```python
from build123d import *

# Parameters (mm, degrees)
CHANFREIN1_SIZE         = 1
CHANFREIN1_SIZE2        = 1.732050808
ESQUISSE3_W             = 48.532957324
ESQUISSE3_H             = 12
ENL_V_MAT_EXTRU_1_DEPTH = 1
ESQUISSE4_OUTSIDE_W     = 40.012
ESQUISSE4_OUTSIDE_H     = 40.012
ESQUISSE4_OUTSIDE_R     = 4.5
ENL_V_MAT_EXTRU_2_DEPTH = 20
ESQUISSE5_W             = 37.366082186
ESQUISSE5_H             = 10
ENL_V_MAT_EXTRU_3_DEPTH = 1.5
CHANFREIN2_SIZE         = 0.5
CHANFREIN3_SIZE         = 0.3


with BuildPart() as part:
    # Esquisse1 → Révolution1 (revolve)
    with BuildSketch(Plane.XY, mode=Mode.PRIVATE) as r_volution1_sk:
        Polygon((5, 73.557112482), (5, -1.442887518), (8.25, -1.442887518), (8.25, -20.442887518), (5, -20.442887518), (5, -31.442887518), (0, -31.442887518), (0, 73.557112482), align=None)
    revolve(r_volution1_sk.sketch.rotate(Axis((0, 73.557112482, 0), (0, -1, 0)), 180), axis=Axis((0, 73.557112482, 0), (0, -1, 0)))  # turned: the seam where the file's is

    # Chanfrein1
    chanfrein1_edges = [part.edges().sort_by_distance(p)[0] for p in [
        (5, -31.442887518, 0),
    ]]
    chanfrein1_side = [part.faces().sort_by_distance(p)[0] for p in [
        (0, -31.442887518, 0),
    ]]
    chamfer(chanfrein1_edges, length=CHANFREIN1_SIZE, length2=CHANFREIN1_SIZE2, reference=chanfrein1_side[0])

    # Esquisse3 → Enlèv. mat.-Extru.1 (cut)
    with BuildSketch(Plane.XY.offset(5)):
        with Locations((0, 37.557112482)):
            Rectangle(ESQUISSE3_W, ESQUISSE3_H)
    extrude(amount=-ENL_V_MAT_EXTRU_1_DEPTH, mode=Mode.SUBTRACT)

    # Esquisse4 outside → Enlèv. mat.-Extru.2 (cut)
    with BuildSketch(Plane(origin=(0, 73.557112482, 0), x_dir=(1, 0, 0), z_dir=(0, 1, 0))):
        Rectangle(ESQUISSE4_OUTSIDE_W, ESQUISSE4_OUTSIDE_H)
        with Locations(Location((0, 0, 0), (0, 0, 180))):  # turned: the seam where the file's is
            Circle(ESQUISSE4_OUTSIDE_R, mode=Mode.SUBTRACT)
    extrude(amount=-ENL_V_MAT_EXTRU_2_DEPTH, mode=Mode.SUBTRACT)

    # Esquisse5 → Enlèv. mat.-Extru.3 (cut)
    with BuildSketch(Plane.XY.offset(5)):
        with Locations((0, 63.557112482)):
            Rectangle(ESQUISSE5_W, ESQUISSE5_H)
    extrude(amount=-ENL_V_MAT_EXTRU_3_DEPTH, mode=Mode.SUBTRACT)

    # Chanfrein2
    chanfrein2_edges = [part.edges().sort_by_distance(p)[0] for p in [
        (4.5, 73.557112482, 0),
    ]]
    chamfer(chanfrein2_edges, length=CHANFREIN2_SIZE)

    # Chanfrein3
    chanfrein3_edges = [part.edges().sort_by_distance(p)[0] for p in [
        (8.25, -1.442887518, 0),
        (8.25, -20.442887518, 0),
    ]]
    chamfer(chanfrein3_edges, length=CHANFREIN3_SIZE)


solid = part.part
```
Input: part model. Units: mm. Frame: model coordinates. A direction names the side the tool comes from. Give positions to 0.01 mm unless a question says otherwise; leave off trailing zeros. Order: outer loops, then holes, each group sorted by start corner. A loop starts at its lowest first (then second) coordinate and runs counter-clockwise, first axis right, second up. Notation, with made-up numbers: (-23, 55) - (28, 55) arc R23 ccw to (28, 91) - close; hole circle Ø3 at (-2.75, 18.25). An arc over 180 degrees is marked (long way). One line per item, written item: value.
1. Reachability of faces 5 (the face through (0, 64, 3.5)), 6 (the face through (0.98, 63.44, -4.39)), 7 (the face through (-5.2, -20.443, -0.1)) from +Z, -Z, +X, -X, +Y, -Y: full face, straight path, thin tool, end or side. Return the list, or none.
Determined:
face 5: +Z, +X, -X
face 6: +Y
face 7: -Y
2. Pin query (flat end, axial travel): pin 1 Ø0.5 at (x, z) = (0.5, 4.5) entering from -Y; pin 2 Ø1 at (x, y) = (-3.5, 8.5) entering from +Z; pin 3 Ø4 at (x, z) = (4, 3.5) entering from +Y; pin 4 Ø8 at (x, y) = (1.5, 18) entering from +Z. Return the tip coordinate at first contact, or that it passes through.
Determined:
pin 1: y = -30.96
pin 2: z = 4
pin 3: y = 73.56
pin 4: z = 5
3. Draft query along Y for faces 1 (the face through (0.651, 25.672, -4.957)), 2 (the face through (0, -31.443, 0)), 3 (the face through (0, 38, 4)), 4 (the face through (5.2, -1.443, -0.1)). Return one class per face: released by +Y, released by -Y, zero draft, split by the parting line, or undercut.
Determined:
face 1: zero draft
face 2: released by -Y
face 3: undercut
face 4: released by +Y
4. Cut plane C-C, the plane y = 15.5. Output: boundary loops of the cut face in (x, z), and give its area (3 significant figures).
Determined:
outline: circle Ø10 at (0, 0)
area: 78.5 mm2
5. Line query: probe 1 along Y at (x, z) = (2.75, 4.25); probe 2 along Z at (x, y) = (0, 16); probe 3 along Z at (x, y) = (-3, -1). Output: solid intervals per line, ascending.
Determined:
probe 1: -20.44 to -1.44
probe 2: -5 to 5
probe 3: -4 to 4
6. Cut plane A-A, the plane z = 0. Output: boundary loops of the cut face in (x, y).
Determined:
outline: (-8.25, -20.14) - (-7.95, -20.44) - (-5, -20.44) - (-5, -29.71) - (-4, -31.44) - (4, -31.44) - (5, -29.71) - (5, -20.44) - (7.95, -20.44) - (8.25, -20.14) - (8.25, -1.74) - (7.95, -1.44) - (5, -1.44) - (5, 53.56) - (4.5, 53.56) - (4.5, 73.06) - (4, 73.56) - (-4, 73.56) - (-4.5, 73.06) - (-4.5, 53.56) - (-5, 53.56) - (-5, -1.44) - (-7.95, -1.44) - (-8.25, -1.74) - close
